Check sheet for the modelled part. Datum: model origin and axes. Units: mm. Round coordinates to 2 decimals unless told otherwise and drop trailing zeros. Loops run counter-clockwise (first coordinate to the right, second up) from the corner with the lowest first, then second, coordinate; pieces in that order, holes last. Notation, with made-up numbers: (23.5, 70) -> (36.5, 70) arc R15 ccw to (36.5, 97) -> close; hole circle Ø8 at (-3.75, -14). An arc over 180 degrees is marked (long way). Use one line per item in the form item = value. Start each with the question number.
(1) Go/stop test with flat-tipped pins: pin 1 (6 mm diameter, centred on y = -50, z = 36.5, fed in from +X); pin 2 (1.5 mm diameter, centred on x = 14, y = -52.5, fed in from -Z); pin 3 (3.5 mm diameter, centred on y = -52, z = -22.5, fed in from -X). Record where each tip stops, or that it passes through.
(2) Sectioned sample at C-C (z = -83). Record the cut outline in (x, y).
(3) Sectioned sample at B-B (x = 1). Record the cut outline in (y, z).
(4) Sectioned sample at A-A (y = -48.25). Record the cut outline in (x, z), and give its area (3 significant figures).
(5) Material ranges on probe 1 along X at (y, z) = (-52.75, 25); probe 2 along X at (y, z) = (-52.5, 31.5), recorded low to high. Write a range as [from, to].
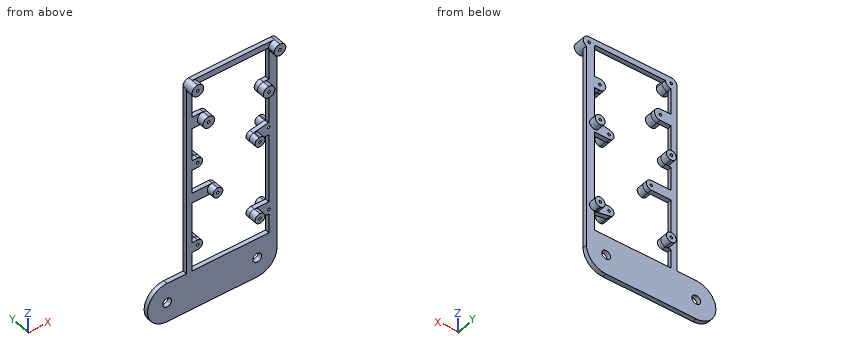
from build123d import *

# Parameters (mm, degrees)
SKETCH2_R                       = 3
SHIFTER_HOLE_IF_DEPTH           = 3
RPI4_SCREW_BOSSES_DEPTH         = 5
RPI4_SCREW_BOSSES_DEPTH_BACK    = 3
SKETCH3_R                       = 3.4
SKETCH3_R_2                     = 0.9
RPI4_SCREW_BOSSES_2_DEPTH       = 5
RPI4_SCREW_BOSSES_2_DEPTH_BACK  = 3
RPI4_SCREW_BOSSES_3_DEPTH       = 5
RPI4_SCREW_BOSSES_3_DEPTH_BACK  = 3
RPI4_SCREW_BOSSES_4_DEPTH       = 5
RPI4_SCREW_BOSSES_4_DEPTH_BACK  = 3
SKETCH4_R                       = 3.4
SKETCH4_R_2                     = 0.9
CAN_SWITCH_SCREW_BOSSES_DEPTH   = 8
CAN_SWITCH_SCREW_BOSSES_2_DEPTH = 8
CAN_SWITCH_SCREW_BOSSES_3_DEPTH = 8
SKETCH5_R                       = 4
SKETCH5_R_2                     = 0.9
F_5V_REG_MOUNT_POSTS_DEPTH      = 8
F_5V_REG_MOUNT_POSTS_2_DEPTH    = 8
F_5V_REG_MOUNT_POSTS_3_DEPTH    = 8
F_5V_REG_MOUNT_POSTS_4_DEPTH    = 8
SKETCH6_R                       = 0.9
IF_LINK_DEPTH                   = 3
CUT_EXTRUDE1_DEPTH              = 125.251760551
CUT_EXTRUDE1_DEPTH_BACK         = 125.251760551


with BuildPart() as part:
    # Sketch2 → SHIFTER HOLE IF (new body)
    with BuildSketch(Plane(origin=(0, -50.5, 0), x_dir=(1, 0, 0), z_dir=(0, 1, 0))):
        with BuildLine():
            Line((-50, 106.5), (12, 106.5))
            ThreePointArc((12, 106.5), (25.5, 93), (12, 79.5))
            Line((12, 79.5), (-50, 79.5))
            ThreePointArc((-50, 79.5), (-63.5, 93), (-50, 106.5))
        make_face()
        with Locations(Location((-50, 93, 0), (0, 0, 270))):
            Circle(SKETCH2_R, mode=Mode.SUBTRACT)
        with Locations(Location((12, 93, 0), (0, 0, 270))):
            Circle(SKETCH2_R, mode=Mode.SUBTRACT)
    extrude(amount=-SHIFTER_HOLE_IF_DEPTH)



with BuildPart() as body_2:
    # Sketch3 → RPI4 SCREW BOSSES (new, two sides: drawn at the far end of the back side and taken through both)
    with BuildSketch(Plane(origin=(0, -50.5, 0), x_dir=(1, 0, 0), z_dir=(0, 1, 0)).offset(-RPI4_SCREW_BOSSES_DEPTH_BACK)):
        with Locations(Location((-29, 63, 0), (0, 0, 270))):
            Circle(SKETCH3_R)
        with Locations(Location((-29, 63, 0), (0, 0, 270))):
            Circle(SKETCH3_R_2, mode=Mode.SUBTRACT)
    extrude(amount=RPI4_SCREW_BOSSES_DEPTH + RPI4_SCREW_BOSSES_DEPTH_BACK)


with BuildPart() as body_3:
    # Sketch3 → RPI4 SCREW BOSSES 2 (new, two sides: drawn at the far end of the back side and taken through both)
    with BuildSketch(Plane(origin=(0, -50.5, 0), x_dir=(1, 0, 0), z_dir=(0, 1, 0)).offset(-RPI4_SCREW_BOSSES_2_DEPTH_BACK)):
        with Locations(Location((20, 63, 0), (0, 0, 270))):
            Circle(SKETCH3_R)
        with Locations(Location((20, 63, 0), (0, 0, 270))):
            Circle(SKETCH3_R_2, mode=Mode.SUBTRACT)
    extrude(amount=RPI4_SCREW_BOSSES_2_DEPTH + RPI4_SCREW_BOSSES_2_DEPTH_BACK)


with BuildPart() as body_4:
    # Sketch3 → RPI4 SCREW BOSSES 3 (new, two sides: drawn at the far end of the back side and taken through both)
    with BuildSketch(Plane(origin=(0, -50.5, 0), x_dir=(1, 0, 0), z_dir=(0, 1, 0)).offset(-RPI4_SCREW_BOSSES_3_DEPTH_BACK)):
        with Locations(Location((20, 5, 0), (0, 0, 270))):
            Circle(SKETCH3_R)
        with Locations(Location((20, 5, 0), (0, 0, 270))):
            Circle(SKETCH3_R_2, mode=Mode.SUBTRACT)
    extrude(amount=RPI4_SCREW_BOSSES_3_DEPTH + RPI4_SCREW_BOSSES_3_DEPTH_BACK)


with BuildPart() as body_5:
    # Sketch3 → RPI4 SCREW BOSSES 4 (new, two sides: drawn at the far end of the back side and taken through both)
    with BuildSketch(Plane(origin=(0, -50.5, 0), x_dir=(1, 0, 0), z_dir=(0, 1, 0)).offset(-RPI4_SCREW_BOSSES_4_DEPTH_BACK)):
        with Locations(Location((-29, 5, 0), (0, 0, 270))):
            Circle(SKETCH3_R)
        with Locations(Location((-29, 5, 0), (0, 0, 270))):
            Circle(SKETCH3_R_2, mode=Mode.SUBTRACT)
    extrude(amount=RPI4_SCREW_BOSSES_4_DEPTH + RPI4_SCREW_BOSSES_4_DEPTH_BACK)


with BuildPart() as body_6:
    # Sketch4 → CAN SWITCH SCREW BOSSES (new body)
    with BuildSketch(Plane(origin=(0, -50.5, 0), x_dir=(1, 0, 0), z_dir=(0, 1, 0))):
        with Locations(Location((10, 61, 0), (0, 0, 270))):
            Circle(SKETCH4_R)
        with Locations(Location((10, 61, 0), (0, 0, 270))):
            Circle(SKETCH4_R_2, mode=Mode.SUBTRACT)
    extrude(amount=-CAN_SWITCH_SCREW_BOSSES_DEPTH)


with BuildPart() as body_7:
    # Sketch4 → CAN SWITCH SCREW BOSSES 2 (new body)
    with BuildSketch(Plane(origin=(0, -50.5, 0), x_dir=(1, 0, 0), z_dir=(0, 1, 0))):
        with Locations(Location((10, 7, 0), (0, 0, 270))):
            Circle(SKETCH4_R)
        with Locations(Location((10, 7, 0), (0, 0, 270))):
            Circle(SKETCH4_R_2, mode=Mode.SUBTRACT)
    extrude(amount=-CAN_SWITCH_SCREW_BOSSES_2_DEPTH)


with BuildPart() as body_8:
    # Sketch4 → CAN SWITCH SCREW BOSSES 3 (new body)
    with BuildSketch(Plane(origin=(0, -50.5, 0), x_dir=(1, 0, 0), z_dir=(0, 1, 0))):
        with Locations(Location((-19, 28, 0), (0, 0, 270))):
            Circle(SKETCH4_R)
        with Locations(Location((-19, 28, 0), (0, 0, 270))):
            Circle(SKETCH4_R_2, mode=Mode.SUBTRACT)
    extrude(amount=-CAN_SWITCH_SCREW_BOSSES_3_DEPTH)


with BuildPart() as body_9:
    # Sketch5 → 5V REG MOUNT POSTS (new body)
    with BuildSketch(Plane(origin=(0, -50.5, 0), x_dir=(1, 0, 0), z_dir=(0, 1, 0))):
        with Locations(Location((-32.75, -51, 0), (0, 0, 270))):
            Circle(SKETCH5_R)
        with Locations(Location((-32.75, -51, 0), (0, 0, 270))):
            Circle(SKETCH5_R_2, mode=Mode.SUBTRACT)
    extrude(amount=-F_5V_REG_MOUNT_POSTS_DEPTH)


with BuildPart() as body_10:
    # Sketch5 → 5V REG MOUNT POSTS 2 (new body)
    with BuildSketch(Plane(origin=(0, -50.5, 0), x_dir=(1, 0, 0), z_dir=(0, 1, 0))):
        with Locations(Location((-25.25, -25, 0), (0, 0, 270))):
            Circle(SKETCH5_R)
        with Locations(Location((-25.25, -25, 0), (0, 0, 270))):
            Circle(SKETCH5_R_2, mode=Mode.SUBTRACT)
    extrude(amount=-F_5V_REG_MOUNT_POSTS_2_DEPTH)


with BuildPart() as body_11:
    # Sketch5 → 5V REG MOUNT POSTS 3 (new body)
    with BuildSketch(Plane(origin=(0, -50.5, 0), x_dir=(1, 0, 0), z_dir=(0, 1, 0))):
        with Locations(Location((16.25, -25, 0), (0, 0, 270))):
            Circle(SKETCH5_R)
        with Locations(Location((16.25, -25, 0), (0, 0, 270))):
            Circle(SKETCH5_R_2, mode=Mode.SUBTRACT)
    extrude(amount=-F_5V_REG_MOUNT_POSTS_3_DEPTH)


with BuildPart() as body_12:
    # Sketch5 → 5V REG MOUNT POSTS 4 (new body)
    with BuildSketch(Plane(origin=(0, -50.5, 0), x_dir=(1, 0, 0), z_dir=(0, 1, 0))):
        with Locations(Location((23.75, -51, 0), (0, 0, 270))):
            Circle(SKETCH5_R)
        with Locations(Location((23.75, -51, 0), (0, 0, 270))):
            Circle(SKETCH5_R_2, mode=Mode.SUBTRACT)
    extrude(amount=-F_5V_REG_MOUNT_POSTS_4_DEPTH)


with BuildPart() as part_1:
    add(part.part)

    add(body_2.part)  # IF LINK merges body 2

    add(body_3.part)  # IF LINK merges body 3

    add(body_4.part)  # IF LINK merges body 4

    add(body_5.part)  # IF LINK merges body 5

    add(body_6.part)  # IF LINK merges body 6

    add(body_7.part)  # IF LINK merges body 7

    add(body_8.part)  # IF LINK merges body 8

    add(body_9.part)  # IF LINK merges body 9

    add(body_10.part)  # IF LINK merges body 10

    add(body_11.part)  # IF LINK merges body 11

    add(body_12.part)  # IF LINK merges body 12
    # Sketch6 → IF LINK (add)
    with BuildSketch(Plane(origin=(0, -50.5, 0), x_dir=(1, 0, 0), z_dir=(0, 1, 0))):
        with BuildLine():
            Line((25.5, 93), (25.5, -47.403126358))
            ThreePointArc((25.5, -47.403126358), (27.647915762, -51.897915762), (23.75, -55))
            Line((23.75, -55), (-32.75, -55))
            ThreePointArc((-32.75, -55), (-35.578427125, -53.828427125), (-36.75, -51))
            Line((-36.75, -51), (-36.75, 79.5))
            Line((-36.75, 79.5), (12, 79.5))
            ThreePointArc((12, 79.5), (21.545941546, 83.454058454), (25.5, 93))
        make_face()
        with Locations(Location((-25.25, -25, 0), (0, 0, 270))):
            Circle(SKETCH6_R, mode=Mode.SUBTRACT)
        with Locations(Location((16.25, -25, 0), (0, 0, 270))):
            Circle(SKETCH6_R, mode=Mode.SUBTRACT)
        with Locations(Location((23.75, -51, 0), (0, 0, 270))):
            Circle(SKETCH6_R, mode=Mode.SUBTRACT)
        with Locations(Location((-32.75, -51, 0), (0, 0, 270))):
            Circle(SKETCH6_R, mode=Mode.SUBTRACT)
        with Locations(Location((-29, 63, 0), (0, 0, 270))):
            Circle(SKETCH6_R, mode=Mode.SUBTRACT)
        with Locations(Location((20, 63, 0), (0, 0, 270))):
            Circle(SKETCH6_R, mode=Mode.SUBTRACT)
        with Locations(Location((10, 61, 0), (0, 0, 270))):
            Circle(SKETCH6_R, mode=Mode.SUBTRACT)
        with Locations(Location((-19, 28, 0), (0, 0, 270))):
            Circle(SKETCH6_R, mode=Mode.SUBTRACT)
        with Locations(Location((10, 7, 0), (0, 0, 270))):
            Circle(SKETCH6_R, mode=Mode.SUBTRACT)
        with Locations(Location((20, 5, 0), (0, 0, 270))):
            Circle(SKETCH6_R, mode=Mode.SUBTRACT)
        with Locations(Location((-29, 5, 0), (0, 0, 270))):
            Circle(SKETCH6_R, mode=Mode.SUBTRACT)
    extrude(amount=-IF_LINK_DEPTH)

    # Sketch7 → Cut-Extrude1 (cut, two sides: drawn at the far end of the back side and taken through both)
    with BuildSketch(Plane(origin=(0, -50.5, 0), x_dir=(1, 0, 0), z_dir=(0, 1, 0)).offset(-CUT_EXTRUDE1_DEPTH_BACK)):
        with BuildLine():
            Line((-32.75, 66.4), (-32.75, 79.5))
            Line((-32.75, 79.5), (20, 79.5))
            Line((20, 79.5), (20, 66.4))
            ThreePointArc((20, 66.4), (19.664972099, 66.383453311), (19.333205141, 66.333974297))
            Line((19.333205141, 66.333974297), (9.333205141, 64.333974297))
            ThreePointArc((9.333205141, 64.333974297), (6.616546689, 60.664972099), (10, 57.6))
            Line((10, 57.6), (20, 57.6))
            Line((20, 57.6), (20, 10.4))
            Line((20, 10.4), (10, 10.4))
            ThreePointArc((10, 10.4), (6.616546689, 7.335027901), (9.333205141, 3.666025703))
            Line((9.333205141, 3.666025703), (19.333205141, 1.666025703))
            ThreePointArc((19.333205141, 1.666025703), (19.664972099, 1.616546689), (20, 1.6))
            Line((20, 1.6), (20, -21))
            Line((20, -21), (16.25, -21))
            ThreePointArc((16.25, -21), (12.25, -25), (16.25, -29))
            Line((16.25, -29), (20, -29))
            Line((20, -29), (20, -49.608058909))
            ThreePointArc((20, -49.608058909), (19.812996063, -50.292893219), (19.75, -51))
            Line((19.75, -51), (-28.75, -51))
            ThreePointArc((-28.75, -51), (-29.921572875, -48.171572875), (-32.75, -47))
            Line((-32.75, -47), (-32.75, -29))
            Line((-32.75, -29), (-25.25, -29))
            ThreePointArc((-25.25, -29), (-21.25, -25), (-25.25, -21))
            Line((-25.25, -21), (-32.75, -21))
            Line((-32.75, -21), (-32.75, 1.6))
            Line((-32.75, 1.6), (-29, 1.6))
            ThreePointArc((-29, 1.6), (-25.6, 5), (-29, 8.4))
            Line((-29, 8.4), (-32.75, 8.4))
            Line((-32.75, 8.4), (-32.75, 24.6))
            Line((-32.75, 24.6), (-19, 24.6))
            ThreePointArc((-19, 24.6), (-15.6, 28), (-19, 31.4))
            Line((-19, 31.4), (-32.75, 31.4))
            Line((-32.75, 31.4), (-32.75, 59.6))
            Line((-32.75, 59.6), (-29, 59.6))
            ThreePointArc((-29, 59.6), (-25.6, 63), (-29, 66.4))
            Line((-29, 66.4), (-32.75, 66.4))
        make_face()
    extrude(amount=CUT_EXTRUDE1_DEPTH + CUT_EXTRUDE1_DEPTH_BACK, mode=Mode.SUBTRACT)


solid = part_1.part
Checks:
q1.pin_1 = 25.5
q1.pin_2 = -106.44
q1.pin_3 = -36.75
q2.outline = (-59.07, -53.5) -> (25.5, -53.5) -> (25.5, -50.5) -> (-59.07, -50.5) -> close
q3.outline = (-53.5, -106.5) -> (-50.5, -106.5) -> (-50.5, -79.5) -> (-53.5, -79.5) -> close; (-53.5, 51) -> (-50.5, 51) -> (-50.5, 55) -> (-53.5, 55) -> close
q4.outline = circle Ø6.8 at (-29, -63); circle Ø6.8 at (-29, -5); circle Ø6.8 at (20, -63); circle Ø6.8 at (20, -5); hole circle Ø1.8 at (-29, -63); hole circle Ø1.8 at (-29, -5); hole circle Ø1.8 at (20, -63); hole circle Ø1.8 at (20, -5)
q4.area = 135 mm2
q5.probe_1 = [-36.75, -26.15], [-24.35, -21.25], [12.25, 15.35], [17.15, 25.5]
q5.probe_2 = [-36.75, -32.75], [20, 25.5]
